Geometry: final body of the model. Coordinates: model frame, mm. Face numbers are marked on the shaded views. A direction names the side the tool comes from. Round coordinates to 2 decimals unless told otherwise and drop trailing zeros. Loops run counter-clockwise (first coordinate to the right, second up) from the corner with the lowest first, then second, coordinate; pieces in that order, holes last. Notation, with made-up numbers: M 47.25,37.5 L 75.25,37.5 A32 ccw 75.25,72.5 Z; hole C 79,11.5 d8. An arc over 180 degrees is marked long. Write each question's results on one line, items separated by ' | '.
```python
from build123d import *

# Parameters (mm, degrees)
F0_W     = 33
F0_H     = 8
F2_R     = 22.125
F3_DEPTH = 25
F5_DEPTH = 7
F7_DEPTH = 8
F8_R     = 4
F9_DEPTH = 25


with BuildPart() as f1:
    # F0 (on Front) → F1 (revolve)
    with BuildSketch(Plane.XZ):
        with Locations((16.5, 4)):
            Rectangle(F0_W, F0_H)
    revolve(axis=Axis((0, 0, 4), (0, 0, 1)))

    # F2 (on Top) → F3 (cut)
    with BuildSketch(Plane.XY):
        Circle(F2_R)
    extrude(amount=F3_DEPTH, mode=Mode.SUBTRACT)

    # F4 (on face) → F5 (cut)
    with BuildSketch(Plane.XY.offset(8)):
        Polygon((-2.5, 22), (0, 22), (2.5, 22), (2.5, 32), (-2.5, 32), align=None)
        Polygon((-14.555569, 28.607436), (-10.728734, 19.368641), (-8.419036, 20.32535), (-6.109337, 21.282058), (-9.936171, 30.520854), align=None)
        Polygon((-24.395184, 20.85965), (-17.324116, 13.788582), (-15.556349, 15.556349), (-13.788582, 17.324116), (-20.85965, 24.395184), align=None)
        Polygon((-30.520854, 9.936171), (-21.282058, 6.109337), (-20.32535, 8.419036), (-19.368641, 10.728734), (-28.607436, 14.555569), align=None)
        Polygon((-32, -2.5), (-22, -2.5), (-22, 0), (-22, 2.5), (-32, 2.5), align=None)
        Polygon((-28.607436, -14.555569), (-19.368641, -10.728734), (-20.32535, -8.419036), (-21.282058, -6.109337), (-30.520854, -9.936171), align=None)
        Polygon((-20.85965, -24.395184), (-13.788582, -17.324116), (-15.556349, -15.556349), (-17.324116, -13.788582), (-24.395184, -20.85965), align=None)
        Polygon((-9.936171, -30.520854), (-6.109337, -21.282058), (-8.419036, -20.32535), (-10.728734, -19.368641), (-14.555569, -28.607436), align=None)
        Polygon((2.5, -32), (2.5, -22), (0, -22), (-2.5, -22), (-2.5, -32), align=None)
        Polygon((14.555569, -28.607436), (10.728734, -19.368641), (8.419036, -20.32535), (6.109337, -21.282058), (9.936171, -30.520854), align=None)
        Polygon((24.395184, -20.85965), (17.324116, -13.788582), (15.556349, -15.556349), (13.788582, -17.324116), (20.85965, -24.395184), align=None)
        Polygon((30.520854, -9.936171), (21.282058, -6.109337), (20.32535, -8.419036), (19.368641, -10.728734), (28.607436, -14.555569), align=None)
        Polygon((32, 2.5), (22, 2.5), (22, 0), (22, -2.5), (32, -2.5), align=None)
        Polygon((28.607436, 14.555569), (19.368641, 10.728734), (20.32535, 8.419036), (21.282058, 6.109337), (30.520854, 9.936171), align=None)
        Polygon((20.85965, 24.395184), (13.788582, 17.324116), (15.556349, 15.556349), (17.324116, 13.788582), (24.395184, 20.85965), align=None)
        Polygon((9.936171, 30.520854), (6.109337, 21.282058), (8.419036, 20.32535), (10.728734, 19.368641), (14.555569, 28.607436), align=None)
    extrude(amount=-F5_DEPTH, mode=Mode.SUBTRACT)

    # F6 (on Top) → F7 (join)
    with BuildSketch(Plane.XY):
        Polygon((43, -5), (43, 0), (43, 5), (32.619013, 5), (32.619013, -5), align=None)
        Polygon((5, 32.619013), (5, 43), (0, 43), (-5, 43), (-5, 32.619013), align=None)
        Polygon((-32.619013, 5), (-43, 5), (-43, 0), (-43, -5), (-32.619013, -5), align=None)
        Polygon((-5, -32.619013), (-5, -43), (0, -43), (5, -43), (5, -32.619013), align=None)
    extrude(amount=F7_DEPTH)

    # F8 (on face) → F9 (cut)
    with BuildSketch(Plane.XY.offset(8)):
        with Locations((0, 37.809506)):
            Circle(F8_R)
        with Locations((37.809506, 0)):
            Circle(F8_R)
        with Locations((-37.809506, 0)):
            Circle(F8_R)
        with Locations((0, -37.809506)):
            Circle(F8_R)
    extrude(amount=-F9_DEPTH, mode=Mode.SUBTRACT)


solid = f1.part
```
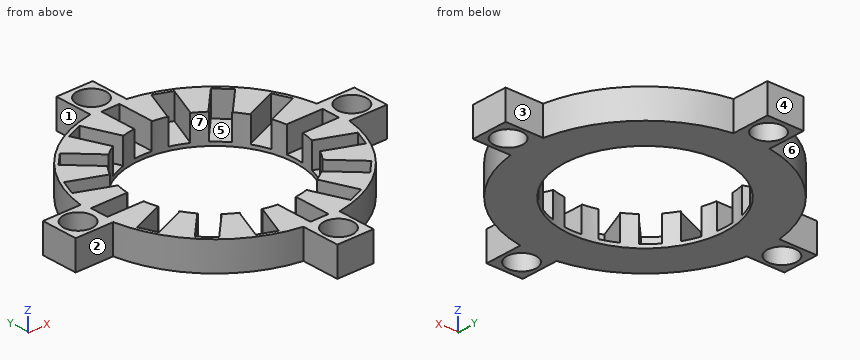
1. Draft query along X for the marked faces 4, 5, 6 and 7. Return one class per face: pulls with the +X half, pulls with the -X half, needs draft (parallel to the pull), parting line crosses it, or undercut.
Answer key:
face 4: needs draft | face 5: undercut | face 6: pulls with the -X half | face 7: undercut
2. Section C-C (y = 16). Output: boundary loops of the cut face in (x, z).
Answer key:
outline: M -28.86,0 L -15.28,0 L -15.28,1 L -19.54,1 L -19.54,8 L -28.86,8 Z; M 15.28,0 L 28.86,0 L 28.86,8 L 19.54,8 L 19.54,1 L 15.28,1 Z
3. Access query for the marked faces 1, 2 and 3. Directions: +Z, -Z, +X, -X, +Y, -Y. A direction counts if a zero-diameter tool reaches every point of the face in a straight line with its end or side. Return the directions, or none.
Answer key:
face 1: +Z, -Z, -X, +Y | face 2: +Z, -Z, -X, -Y | face 3: +Z, -Z, +X, +Y
4. Pin query (flat end, axial travel): P1, Ø6.5, axis at x = 37.81, y = 0, coming from the -Z side; P2, Ø1, axis at x = -12.5, z = 1, coming from the +Y side; P3, Ø1, axis at x = -24, z = 3.5, coming from the +Y side; P4, Ø2, axis at x = -28.5, z = 3, coming from the +Y side. Return the tip coordinate at first contact, or that it passes through.
Answer key:
P1: passes through | P2: stops at y = 30.74 | P3: stops at y = 23.17 | P4: stops at y = 18.24
5. Section A-A (y = 0). Output: boundary loops of the cut face in (x, z) (1 decimal), then the cut area to 4 significant figures.
Answer key:
outline: M -43,0 L -41.8,0 L -41.8,8 L -43,8 Z; M -33.8,0 L -22.1,0 L -22.1,1 L -32,1 L -32,8 L -33.8,8 Z; M 22.1,0 L 33.8,0 L 33.8,8 L 32,8 L 32,1 L 22.1,1 Z; M 41.8,0 L 43,0 L 43,8 L 41.8,8 Z | area: 67.75 mm²
6. Ray query, probe 1 along Y at (x, z) = (0, 5); probe 2 along X at (y, z) = (1.5, 0.5); probe 3 along Y at (x, z) = (11.5, 7). Return the intervals inside material, ascending.
Answer key:
probe 1: y = -43 to -41.81, -33.81 to -32, 32 to 33.81, 41.81 to 43 | probe 2: x = -43 to -41.52, -34.1 to -22.07, 22.07 to 34.1, 41.52 to 43 | probe 3: y = -30.93 to -29.87, -21.23 to -18.9, 18.9 to 21.23, 29.87 to 30.93
7. Section B-B (x = 36.5). Output: boundary loops of the cut face in (y, z).
Answer key:
outline: M -5,0 L -3.78,0 L -3.78,8 L -5,8 Z; M 3.78,0 L 5,0 L 5,8 L 3.78,8 Z
